Can you work these out from the model? Positions are in its coordinate system, mm. Face numbers are marked on the shaded views. Coordinates: 2 decimals unless noted, no trailing zeros. Order: outer loops, then holes, each group sorted by start corner. A loop starts at its lowest first (then second) coordinate and runs counter-clockwise, first axis right, second up. Notation, with made-up numbers: (32, 80.25) -> (71, 80.25) arc R13 ccw to (71, 84.25) -> close; hole circle Ø2 at (-18, 11). An arc over 180 degrees is marked (long way). Answer in a Markdown table with one row per item.
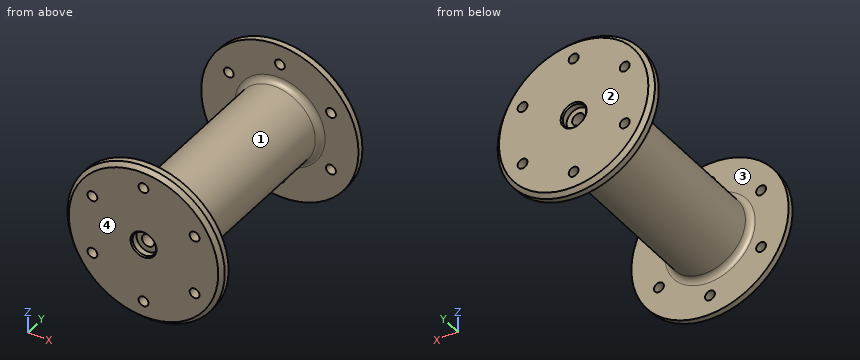
```python
from build123d import *

# Parameters (mm, degrees)
SKETCH1_R                = 20
BOSS_EXTRUDE1_DEPTH      = 50
SKETCH2_R                = 40
BOSS_EXTRUDE2_DEPTH      = 5
CHAMFER1_SIZE            = 2
CUT_EXTRUDE1_START       = -295
SKETCH3_R                = 2.5
CUT_EXTRUDE1_DEPTH       = 690
CIRPATTERN1_COUNT        = 6
FILLET1_R                = 3
CUT_EXTRUDE2_START       = -102.4186
SKETCH6_R                = 3.125
CUT_EXTRUDE2_DEPTH       = 107
CHAMFER1_OF_MIRROR3_SIZE = 2
FILLET1_OF_MIRROR3_R     = 3
MIRROR4_START            = -295
MIRROR4_COPY_1_SKETCH_R  = 2.5
MIRROR4_COPY_1_DEPTH     = 690
MIRROR4_COPY_2_SKETCH_R  = 2.5
MIRROR4_COPY_2_DEPTH     = 690
MIRROR4_COPY_3_SKETCH_R  = 2.5
MIRROR4_COPY_3_DEPTH     = 690
MIRROR4_COPY_4_SKETCH_R  = 2.5
MIRROR4_COPY_4_DEPTH     = 690
MIRROR4_COPY_5_SKETCH_R  = 2.5
MIRROR4_COPY_5_DEPTH     = 690


with BuildPart() as part:
    # Sketch1 → Boss-Extrude1 (new body, symmetric)
    with BuildSketch(Plane(origin=(0, 0, 0), x_dir=(1, 0, 0), z_dir=(0, 1, 0))):
        Circle(SKETCH1_R)
    extrude(amount=BOSS_EXTRUDE1_DEPTH, both=True)

    # Sketch2 → Boss-Extrude2 (add)
    with BuildSketch(Plane(origin=(0, 50, 0), x_dir=(1, 0, 0), z_dir=(0, 1, 0))):
        Circle(SKETCH2_R)
    boss_extrude2 = extrude(amount=BOSS_EXTRUDE2_DEPTH)

    # Chamfer1
    chamfer1_edges = [part.edges().sort_by_distance(p)[0] for p in [
        (-40, 55, 0),
    ]]
    chamfer(chamfer1_edges, length=CHAMFER1_SIZE)

    # Sketch3 → Cut-Extrude1 (cut)
    with BuildSketch(Plane(origin=(0, 55, 0), x_dir=(1, 0, 0), z_dir=(0, 1, 0)).offset(CUT_EXTRUDE1_START)):
        with Locations((0, 30)):
            Circle(SKETCH3_R)
    cut_extrude1 = extrude(amount=CUT_EXTRUDE1_DEPTH, mode=Mode.SUBTRACT)

    # CirPattern1: Cut-Extrude1 ×6 about axis
    cirpattern1_axis = Axis((0, 0, 0), (0, 1, 0))
    for i in range(1, CIRPATTERN1_COUNT):
        add(cut_extrude1.rotate(cirpattern1_axis, i * 360 / CIRPATTERN1_COUNT), mode=Mode.SUBTRACT)

    # Fillet1
    fillet1_edges = [part.edges().sort_by_distance(p)[0] for p in [
        (-20, 50, 0),
    ]]
    fillet(fillet1_edges, radius=FILLET1_R)

    # Sketch5 → CBORE for #12 Binding Head Machine Screw1 (revolve, cut)
    with BuildSketch(Plane(origin=(0, 55, 0), x_dir=(0, 0, 1), z_dir=(1, 0, 0))):
        Polygon((0, 0), (0, 1.927208746), (3.1242, 0.05), (3.1242, 3.5814), (5.95376, 3.5814), (5.95376, 0.635), (6.58876, 0), align=None)
    cbore_for_12_binding_head_machine_screw = revolve(axis=Axis((0, 61.35, 0), (0, -1, 0)), mode=Mode.SUBTRACT)

    # Sketch6 → Cut-Extrude2 (cut)
    with BuildSketch(Plane(origin=(0, 51.4186, 0), x_dir=(1, 0, 0), z_dir=(0, 1, 0)).offset(CUT_EXTRUDE2_START)):
        Circle(SKETCH6_R)
    cut_extrude2 = extrude(amount=CUT_EXTRUDE2_DEPTH, mode=Mode.SUBTRACT)

    # Mirror3: Boss-Extrude2, CBORE for #12 Binding Head Machine Screw1, Cut-Extrude2 across plane
    add(boss_extrude2.mirror(Plane.ZX))
    add(cbore_for_12_binding_head_machine_screw.mirror(Plane.ZX), mode=Mode.SUBTRACT)
    add(cut_extrude2.mirror(Plane.ZX), mode=Mode.SUBTRACT)

    # Chamfer1 of Mirror3
    chamfer1_of_mirror3_edges = [part.edges().sort_by_distance(p)[0] for p in [
        (-40, -55, 0),
    ]]
    chamfer(chamfer1_of_mirror3_edges, length=CHAMFER1_OF_MIRROR3_SIZE)

    # Fillet1 of Mirror3
    fillet1_of_mirror3_edges = [part.edges().sort_by_distance(p)[0] for p in [
        (-20, -50, 0),
    ]]
    fillet(fillet1_of_mirror3_edges, radius=FILLET1_OF_MIRROR3_R)

    # Mirror4: Cut-Extrude1 across plane
    add(cut_extrude1.mirror(Plane.ZX), mode=Mode.SUBTRACT)

    # Mirror4 copy 1 sketch → Mirror4 copy 1 (cut)
    with BuildSketch(Plane(origin=(0, -55, 0), x_dir=(0.5, 0, -0.866025404), z_dir=(0, -1, 0)).offset(MIRROR4_START)):
        with Locations((0, -30)):
            Circle(MIRROR4_COPY_1_SKETCH_R)
    extrude(amount=MIRROR4_COPY_1_DEPTH, mode=Mode.SUBTRACT)

    # Mirror4 copy 2 sketch → Mirror4 copy 2 (cut)
    with BuildSketch(Plane(origin=(0, -55, 0), x_dir=(-0.5, 0, -0.866025404), z_dir=(0, -1, 0)).offset(MIRROR4_START)):
        with Locations((0, -30)):
            Circle(MIRROR4_COPY_2_SKETCH_R)
    extrude(amount=MIRROR4_COPY_2_DEPTH, mode=Mode.SUBTRACT)

    # Mirror4 copy 3 sketch → Mirror4 copy 3 (cut)
    with BuildSketch(Plane(origin=(0, -55, 0), x_dir=(-1, 0, 0), z_dir=(0, -1, 0)).offset(MIRROR4_START)):
        with Locations((0, -30)):
            Circle(MIRROR4_COPY_3_SKETCH_R)
    extrude(amount=MIRROR4_COPY_3_DEPTH, mode=Mode.SUBTRACT)

    # Mirror4 copy 4 sketch → Mirror4 copy 4 (cut)
    with BuildSketch(Plane(origin=(0, -55, 0), x_dir=(-0.5, 0, 0.866025404), z_dir=(0, -1, 0)).offset(MIRROR4_START)):
        with Locations((0, -30)):
            Circle(MIRROR4_COPY_4_SKETCH_R)
    extrude(amount=MIRROR4_COPY_4_DEPTH, mode=Mode.SUBTRACT)

    # Mirror4 copy 5 sketch → Mirror4 copy 5 (cut)
    with BuildSketch(Plane(origin=(0, -55, 0), x_dir=(0.5, 0, 0.866025404), z_dir=(0, -1, 0)).offset(MIRROR4_START)):
        with Locations((0, -30)):
            Circle(MIRROR4_COPY_5_SKETCH_R)
    extrude(amount=MIRROR4_COPY_5_DEPTH, mode=Mode.SUBTRACT)


solid = part.part
```
(1) Will these pins go through, and if not, where does the flat tip stop? pin 1 Ø5 at (x, z) = (0, 0) entering from +Y; pin 2 Ø7 at (x, z) = (0, 0) entering from -Y; pin 3 Ø12 at (y, z) = (39.5, -9) entering from -X; pin 4 Ø1 at (y, z) = (-17, 3) entering from +X.
Response values:
| item | result |
|---|---|
| pin 1 | through |
| pin 2 | y = -51.42 |
| pin 3 | x = -19.77 |
| pin 4 | x = 19.84 |
(2) Suppose I cut it at B-B (y = 9). Please give me the cut outline in (x, z) (3 decimals).
Response values:
| item | result |
|---|---|
| outline | circle Ø40 at (0, 0); hole circle Ø6.25 at (0, 0) |
(3) I need wall thicknesses on line 1 (Z direction, x = 0, y = 52.8); line 2 (Y direction, x = 21, z = 15.5); line 3 (X direction, y = 53, z = 0). Which ranges of each line are inside material? Lowest first, please. Write a range as [from, to].
Response values:
| item | result |
|---|---|
| line 1 | [-40, -32.5], [-27.5, -5.95], [5.95, 27.5], [32.5, 40] |
| line 2 | [-55, -50], [50, 55] |
| line 3 | [-40, -5.95], [5.95, 40] |
(4) Suppose I cut it at A-A (x = 0). Count the separate pieces of the cut face and the enclosed holes in it, and give its area (3 significant figures).
Response values:
| item | result |
|---|---|
| separate pieces | 6 |
| enclosed holes | 0 |
| area | 3,970 mm2 |
(5) We'd pull the mould along Y, two halves only. Please class the marked faces 1, 2, 3 and 4: +Y half, -Y half, draft (parallel to the pull), parting line (faces both ways), or undercut.
Response values:
| item | result |
|---|---|
| face 1 | undercut |
| face 2 | +Y half |
| face 3 | undercut |
| face 4 | -Y half |
